from build123d import *

# Parameters (mm, degrees)
BR_EXTRUDE_DEPTH      = 122.5
BR_EXTRUDE_DEPTH_BACK = 77.5


with BuildPart() as part:
    # Sketch2 → BR_Extrude (new body, two sides)
    with BuildSketch(Plane(origin=(0, 0, 0), x_dir=(0, 0, -1), z_dir=(1, 0, 0))) as br_extrude_sk:
        with BuildLine():
            Line((-10.05, 11.676345597), (-10.05, 16.5))
            Line((-10.05, 16.5), (-5, 16.5))
            Line((-5, 16.5), (-5, 21))
            Line((-5, 21), (-5.8, 21))
            Line((-5.8, 21), (-5.8, 22.5))
            Line((-5.8, 22.5), (-19.5, 22.5))
            ThreePointArc((-19.5, 22.5), (-21.621320344, 21.621320344), (-22.5, 19.5))
            Line((-22.5, 19.5), (-22.5, 5.8))
            Line((-22.5, 5.8), (-21, 5.8))
            Line((-21, 5.8), (-21, 5))
            Line((-21, 5), (-16.5, 5))
            Line((-16.5, 5), (-16.5, 10.05))
            Line((-16.5, 10.05), (-11.676345597, 10.05))
            Line((-11.676345597, 10.05), (-6.411275155, 4.784929559))
            ThreePointArc((-6.411275155, 4.784929559), (-8, 0), (-6.411275155, -4.784929559))
            Line((-6.411275155, -4.784929559), (-11.676345597, -10.05))
            Line((-11.676345597, -10.05), (-16.5, -10.05))
            Line((-16.5, -10.05), (-16.5, -5))
            Line((-16.5, -5), (-21, -5))
            Line((-21, -5), (-21, -5.8))
            Line((-21, -5.8), (-22.5, -5.8))
            Line((-22.5, -5.8), (-22.5, -19.5))
            ThreePointArc((-22.5, -19.5), (-21.621320344, -21.621320344), (-19.5, -22.5))
            Line((-19.5, -22.5), (-5.8, -22.5))
            Line((-5.8, -22.5), (-5.8, -21))
            Line((-5.8, -21), (-5, -21))
            Line((-5, -21), (-5, -16.5))
            Line((-5, -16.5), (-10.05, -16.5))
            Line((-10.05, -16.5), (-10.05, -11.676345597))
            Line((-10.05, -11.676345597), (-4.784929559, -6.411275155))
            ThreePointArc((-4.784929559, -6.411275155), (0, -8), (4.784929559, -6.411275155))
            Line((4.784929559, -6.411275155), (10.05, -11.676345597))
            Line((10.05, -11.676345597), (10.05, -16.5))
            Line((10.05, -16.5), (5, -16.5))
            Line((5, -16.5), (5, -21))
            Line((5, -21), (5.8, -21))
            Line((5.8, -21), (5.8, -22.5))
            Line((5.8, -22.5), (19.5, -22.5))
            ThreePointArc((19.5, -22.5), (21.621320344, -21.621320344), (22.5, -19.5))
            Line((22.5, -19.5), (22.5, -5.8))
            Line((22.5, -5.8), (21, -5.8))
            Line((21, -5.8), (21, -5))
            Line((21, -5), (16.5, -5))
            Line((16.5, -5), (16.5, -10.05))
            Line((16.5, -10.05), (11.676345597, -10.05))
            Line((11.676345597, -10.05), (6.411275155, -4.784929559))
            ThreePointArc((6.411275155, -4.784929559), (8, 0), (6.411275155, 4.784929559))
            Line((6.411275155, 4.784929559), (11.676345597, 10.05))
            Line((11.676345597, 10.05), (16.5, 10.05))
            Line((16.5, 10.05), (16.5, 5))
            Line((16.5, 5), (21, 5))
            Line((21, 5), (21, 5.8))
            Line((21, 5.8), (22.5, 5.8))
            Line((22.5, 5.8), (22.5, 19.5))
            ThreePointArc((22.5, 19.5), (21.621320344, 21.621320344), (19.5, 22.5))
            Line((19.5, 22.5), (5.8, 22.5))
            Line((5.8, 22.5), (5.8, 21))
            Line((5.8, 21), (5, 21))
            Line((5, 21), (5, 16.5))
            Line((5, 16.5), (10.05, 16.5))
            Line((10.05, 16.5), (10.05, 11.676345597))
            Line((10.05, 11.676345597), (4.784929559, 6.411275155))
            ThreePointArc((4.784929559, 6.411275155), (0, 8), (-4.784929559, 6.411275155))
            Line((-4.784929559, 6.411275155), (-10.05, 11.676345597))
        make_face()
        with BuildLine():
            Line((11.55, 11.55), (11.55, 18))
            Line((11.55, 18), (7.5, 18))
            Line((7.5, 18), (7.5, 21))
            Line((7.5, 21), (18.5, 21))
            ThreePointArc((18.5, 21), (20.267766953, 20.267766953), (21, 18.5))
            Line((21, 18.5), (21, 7.5))
            Line((21, 7.5), (18, 7.5))
            Line((18, 7.5), (18, 11.55))
            Line((18, 11.55), (11.55, 11.55))
        make_face(mode=Mode.SUBTRACT)
        with BuildLine():
            Line((11.55, -11.55), (18, -11.55))
            Line((18, -11.55), (18, -7.5))
            Line((18, -7.5), (21, -7.5))
            Line((21, -7.5), (21, -18.5))
            ThreePointArc((21, -18.5), (20.267766953, -20.267766953), (18.5, -21))
            Line((18.5, -21), (7.5, -21))
            Line((7.5, -21), (7.5, -18))
            Line((7.5, -18), (11.55, -18))
            Line((11.55, -18), (11.55, -11.55))
        make_face(mode=Mode.SUBTRACT)
        with BuildLine():
            Line((-11.55, 11.55), (-18, 11.55))
            Line((-18, 11.55), (-18, 7.5))
            Line((-18, 7.5), (-21, 7.5))
            Line((-21, 7.5), (-21, 18.5))
            ThreePointArc((-21, 18.5), (-20.267766953, 20.267766953), (-18.5, 21))
            Line((-18.5, 21), (-7.5, 21))
            Line((-7.5, 21), (-7.5, 18))
            Line((-7.5, 18), (-11.55, 18))
            Line((-11.55, 18), (-11.55, 11.55))
        make_face(mode=Mode.SUBTRACT)
        with BuildLine():
            Line((-11.55, -11.55), (-11.55, -18))
            Line((-11.55, -18), (-7.5, -18))
            Line((-7.5, -18), (-7.5, -21))
            Line((-7.5, -21), (-18.5, -21))
            ThreePointArc((-18.5, -21), (-20.267766953, -20.267766953), (-21, -18.5))
            Line((-21, -18.5), (-21, -7.5))
            Line((-21, -7.5), (-18, -7.5))
            Line((-18, -7.5), (-18, -11.55))
            Line((-18, -11.55), (-11.55, -11.55))
        make_face(mode=Mode.SUBTRACT)
        with BuildLine():
            Line((-6.007327293, -1.059253884), (-4.924038765, -0.868240888))
            ThreePointArc((-4.924038765, -0.868240888), (-5, 0), (-4.924038765, 0.868240888))
            Line((-4.924038765, 0.868240888), (-6.007327293, 1.059253884))
            ThreePointArc((-6.007327293, 1.059253884), (-5.635665148, 2.334368937), (-4.99682747, 3.498816262))
            Line((-4.99682747, 3.498816262), (-4.095760221, 2.867882182))
            ThreePointArc((-4.095760221, 2.867882182), (-3.535533906, 3.535533906), (-2.867882182, 4.095760221))
            Line((-2.867882182, 4.095760221), (-3.498816262, 4.99682747))
            ThreePointArc((-3.498816262, 4.99682747), (-2.334368937, 5.635665148), (-1.059253884, 6.007327293))
            Line((-1.059253884, 6.007327293), (-0.868240888, 4.924038765))
            ThreePointArc((-0.868240888, 4.924038765), (0, 5), (0.868240888, 4.924038765))
            Line((0.868240888, 4.924038765), (1.059253884, 6.007327293))
            ThreePointArc((1.059253884, 6.007327293), (2.334368937, 5.635665148), (3.498816262, 4.99682747))
            Line((3.498816262, 4.99682747), (2.867882182, 4.095760221))
            ThreePointArc((2.867882182, 4.095760221), (3.535533906, 3.535533906), (4.095760221, 2.867882182))
            Line((4.095760221, 2.867882182), (4.99682747, 3.498816262))
            ThreePointArc((4.99682747, 3.498816262), (5.635665148, 2.334368937), (6.007327293, 1.059253884))
            Line((6.007327293, 1.059253884), (4.924038765, 0.868240888))
            ThreePointArc((4.924038765, 0.868240888), (5, 0), (4.924038765, -0.868240888))
            Line((4.924038765, -0.868240888), (6.007327293, -1.059253884))
            ThreePointArc((6.007327293, -1.059253884), (5.635665148, -2.334368937), (4.99682747, -3.498816262))
            Line((4.99682747, -3.498816262), (4.095760221, -2.867882182))
            ThreePointArc((4.095760221, -2.867882182), (3.535533906, -3.535533906), (2.867882182, -4.095760221))
            Line((2.867882182, -4.095760221), (3.498816262, -4.99682747))
            ThreePointArc((3.498816262, -4.99682747), (2.334368937, -5.635665148), (1.059253884, -6.007327293))
            Line((1.059253884, -6.007327293), (0.868240888, -4.924038765))
            ThreePointArc((0.868240888, -4.924038765), (0, -5), (-0.868240888, -4.924038765))
            Line((-0.868240888, -4.924038765), (-1.059253884, -6.007327293))
            ThreePointArc((-1.059253884, -6.007327293), (-2.334368937, -5.635665148), (-3.498816262, -4.99682747))
            Line((-3.498816262, -4.99682747), (-2.867882182, -4.095760221))
            ThreePointArc((-2.867882182, -4.095760221), (-3.535533906, -3.535533906), (-4.095760221, -2.867882182))
            Line((-4.095760221, -2.867882182), (-4.99682747, -3.498816262))
            ThreePointArc((-4.99682747, -3.498816262), (-5.635665148, -2.334368937), (-6.007327293, -1.059253884))
        make_face(mode=Mode.SUBTRACT)
    extrude(amount=BR_EXTRUDE_DEPTH)
    extrude(br_extrude_sk.sketch, amount=-BR_EXTRUDE_DEPTH_BACK)


solid = part.part
Geometry: final body of the model. Coordinates: model frame, mm. A direction names the side the tool comes from. Give positions to 0.01 mm unless a question says otherwise; leave off trailing zeros. Loops run counter-clockwise (first coordinate to the right, second up) from the corner with the lowest first, then second, coordinate; pieces in that order, holes last. Notation, with made-up numbers: M 51,28 L 68,28 A27 ccw 68,50 Z; hole C 69.5,-38.75 d2. An arc over 180 degrees is marked long. Put each result on its own line as item: value. Start each with the question number.
1) Pull-direction query (Y, two-part tool) for faces 1 (the flat face through (24, -13, 22.5)), 2 (the flat face through (24, -10.05, 14)), 3 (the flat face through (24, 22.5, -13)); classes: pulls with the +Y half, pulls with the -Y half, needs draft (parallel to the pull), parting line crosses it, or undercut.
2) Cut plane C-C (x = 48.5). Give the number of separate pieces and of enclosed holes in the cut face, then the cut area to 3 significant figures.
3) Access query for faces 4 (the flat face through (24, 19, -5)), 5 (the flat face through (24, 16.5, -7)), 6 (the flat face through (24, -19, -5)). Directions: +Z, -Z, +X, -X, +Y, -Y. A direction counts if a zero-diameter tool reaches every point of the face in a straight line with its end or side. Return the directions, or none.
4) Contact query for flat-ended pins moving along their axis: pin 1 (2 mm diameter, centred on x = 35.5, z = 0.5, fed in from -Y); pin 2 (1.6 mm diameter, centred on x = -10.5, y = 21.5, fed in from +Z). Output: stop coordinate, or through.
5) Ray query, line 1 along Y through (x, z) = (-35, 14); line 2 along Z through (x, y) = (36, -18.5). Return the intervals inside material, ascending.
6) Cut plane A-A (y = -14). Output: boundary loops of the cut face in (x, z), then the cut area to 3 significant figures.
Verdict:
1. face 1: needs draft
1. face 2: undercut
1. face 3: pulls with the +Y half
2. separate pieces: 1
2. enclosed holes: 5
2. area: 560 mm2
3. face 4: +X, -X, +Y
3. face 5: +X, -X
3. face 6: +X, -X, -Y
4. pin 1: y = -8
4. pin 2: z = 22.25
5. line 1: -22.5 to -21, -11.55 to -10.05, 10.05 to 11.55, 21 to 22.5
5. line 2: -22.5 to -21, -7.5 to -5, 5 to 7.5, 21 to 22.5
6. outline: M -77.5,-22.5 L 122.5,-22.5 L 122.5,-21 L -77.5,-21 Z; M -77.5,-11.55 L 122.5,-11.55 L 122.5,-10.05 L -77.5,-10.05 Z; M -77.5,10.05 L 122.5,10.05 L 122.5,11.55 L -77.5,11.55 Z; M -77.5,21 L 122.5,21 L 122.5,22.5 L -77.5,22.5 Z
6. area: 1,200 mm2
